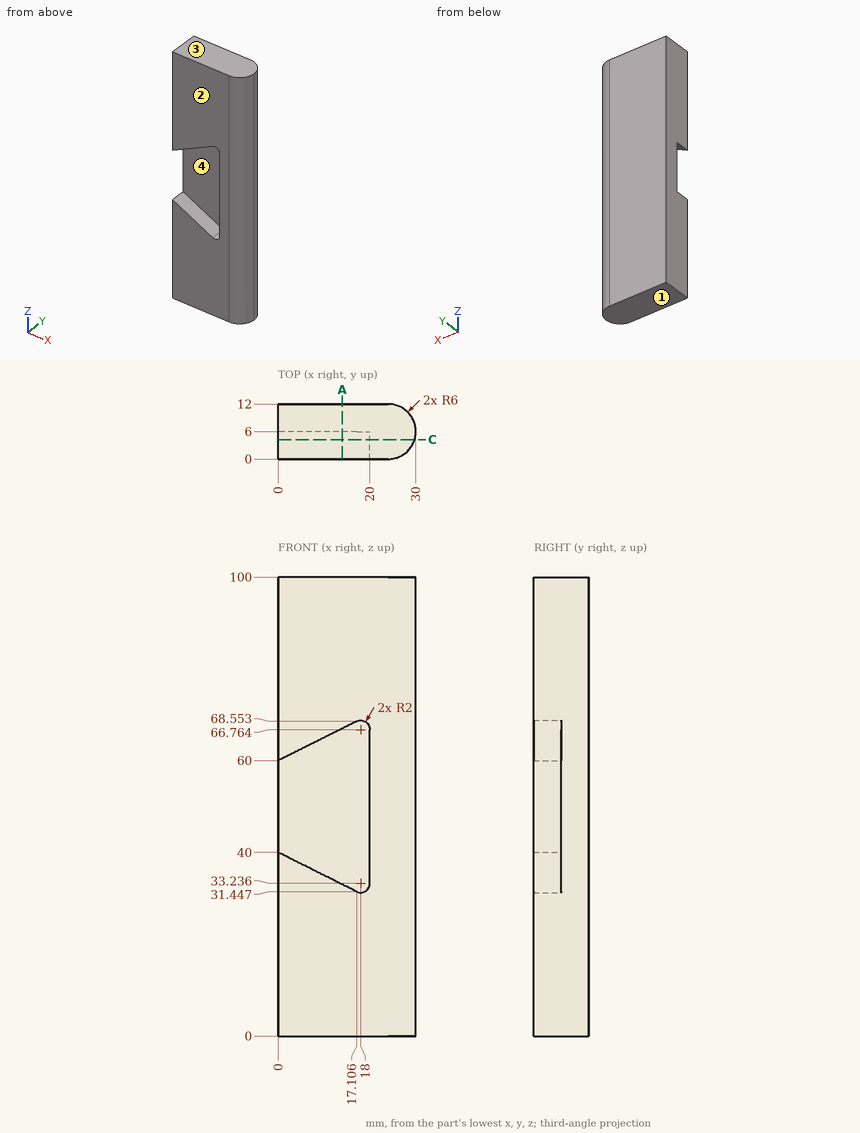
Geometry: see drawing. Coordinates: mm, zero at the bounding-box minimum. Give positions to 0.01 mm unless a question says otherwise; leave off trailing zeros. Loops run counter-clockwise (first coordinate to the right, second up) from the corner with the lowest first, then second, coordinate; pieces in that order, holes last. Notation, with made-up numbers: (-3.75, 38.5) -> (4.25, 38.5) arc R20 ccw to (4.25, 76.5) -> close; hole circle Ø9 at (82, 59.25). An arc over 180 degrees is marked (long way). Use CSV: the item, a comma, the result in double quotes.
(1) Pull-direction query (Z, two-part tool) for the marked faces 1, 2, 3 and 4; classes: released by +Z, released by -Z, zero draft, split by the parting line, or undercut.
From the geometry:
face 1,"released by -Z"
face 2,"zero draft"
face 3,"released by +Z"
face 4,"undercut"
(2) First-contact query: P1, Ø2, axis at x = 14.5, z = 56, coming from the -Y side; P2, Ø1.8, axis at y = 4, z = 51, coming from the -X side. Flat tips, straight axial feed; report the tip coordinate or a pass-through.
From the geometry:
P1,"y = 6"
P2,"x = 20"
(3) Ray query, line 1 along Z through (x, y) = (7.5, 3); line 2 along Z through (x, y) = (16.5, 1.25); line 3 along X through (y, z) = (5.5, 89.5). Return the intervals inside material, ascending. Write a range as [from, to].
From the geometry:
line 1,"[0, 36.25], [63.75, 100]"
line 2,"[0, 31.75], [68.25, 100]"
line 3,"[0, 29.98]"
(4) Cut plane C-C (y = 4.25). Output: boundary loops of the cut face in (x, z) (1 decimal).
From the geometry:
outline,"(0, 0) -> (29.7, 0) -> (29.7, 100) -> (0, 100) -> (0, 60) -> (17.1, 68.6) arc R2 cw to (20, 66.8) -> (20, 33.2) arc R2 cw to (17.1, 31.4) -> (0, 40) -> close"
(5) Cut plane A-A (x = 14). Output: boundary loops of the cut face in (y, z), plus the area to 3 significant figures.
From the geometry:
outline,"(0, 0) -> (12, 0) -> (12, 100) -> (0, 100) -> (0, 67) -> (6, 67) -> (6, 33) -> (0, 33) -> close"
area,"996 mm^2"
